Read the model definition and answer for the solid it produces. Units are mm, in the model's axes. A direction names the side the tool comes from. Give positions to 0.01 mm unless a question says otherwise; leave off trailing zeros. Order: outer loops, then holes, each group sorted by start corner. A loop starts at its lowest first (then second) coordinate and runs counter-clockwise, first axis right, second up. Notation, with made-up numbers: (20, 71) -> (61, 71) arc R21 cw to (61, 103) -> close; hole circle Ø7 at (64.5, -34). An arc over 180 degrees is marked (long way). Answer as CSV lines item,"result". Start each with the question number.
1) Straight lines are drawn through the part: L1, parallel to Z at x = 19.5, y = 1.7; L2, parallel to Z at x = 19.25, y = 1.35; L3, parallel to X at y = 0.4, z = 3. For each, find the intervals that lie inside material, in ascending order. Write a range as from..to.
2) Find section B-B (z = 2). Determine the outline of the cut face in (x, y), and give its area (3 significant figures).
3) For faces 1 (the face through (14, 2, 0)), 2 (the face through (19, 2, -3)), 3 (the face through (9, 1, 2.5)), determine the directions among +Z, -Z, +X, -X, +Y, -Y from which every point of the face is accessible in a straight line to the end or side of a thin tool.
4) Flat-ended cylindrical pins translate along their axes: pin 1 Ø1.5 at (x, y) = (10, 1.5) entering from -Z; pin 2 Ø0.6 at (x, y) = (11.5, 1) entering from -Z; pin 3 Ø0.9 at (y, z) = (2, -2) entering from +X. Find the tip coordinate at first contact, or state that the pin passes through.
5) Find section C-C (x = 5.75). Determine the outline of the cut face in (y, z).
6) Find section D-D (y = 1.8). State how many separate pieces and enclosed holes the cut face has, and give its area (3 significant figures).
7) The mould has two halves that part along X. Classify faces 4 (the face through (8.328, 1, 4)), 5 (the face through (13, 1, 2.5)), 6 (the face through (15, 0, 12)), 7 (the face through (24.4, 1.52, 26.43)): +X half, -X half, draft (parallel to the pull), parting line (faces both ways), or undercut.
8) Find section A-A (z = 8). Determine the outline of the cut face in (x, y), and give its area (3 significant figures).
```python
from build123d import *

# Parameters (mm, degrees)
SKETCH_1_W          = 25
SKETCH_1_H          = 5
EXTRUDE_1_DEPTH     = 24
SKETCH_2_W          = 5
SKETCH_2_H          = 5
SKETCH_2_W_2        = 8
EXTRUDE_2_DEPTH     = 3
CUT_EXTRUDE_2_DEPTH = 5
EXTRUDE_3_DEPTH     = 5
FILLET_1_R          = 5
FILLET_2_R          = 2
CUT_EXTRUDE_4_DEPTH = 2
CUT_EXTRUDE_5_DEPTH = 3
SKETCH_9_R          = 2
CUT_EXTRUDE_6_DEPTH = 3
SKETCH_10_W         = 7
SKETCH_10_H         = 3
CUT_EXTRUDE_7_DEPTH = 3


with BuildPart() as part:
    # 草图1 → 凸台-拉伸1 (new body)
    with BuildSketch(Plane.XY):
        with Locations((12.5, 2.5)):
            Rectangle(SKETCH_1_W, SKETCH_1_H)
    extrude(amount=EXTRUDE_1_DEPTH)

    # 草图2 → 凸台-拉伸2 (add)
    with BuildSketch(Plane(origin=(0, 0, 0), x_dir=(-1, 0, 0), z_dir=(0, 0, -1))):
        with Locations((-4.5, 2.5)):
            Rectangle(SKETCH_2_W, SKETCH_2_H)
        with Locations((-19, 2.5)):
            Rectangle(SKETCH_2_W_2, SKETCH_2_H)
    extrude(amount=EXTRUDE_2_DEPTH)

    # 草图3 → 切除-拉伸2 (cut)
    with BuildSketch(Plane.XZ):
        Polygon((12.5, 24), (0, 24), (0, 0), align=None)
    extrude(amount=-CUT_EXTRUDE_2_DEPTH, mode=Mode.SUBTRACT)

    # 草图4 → 凸台-拉伸3 (add)
    with BuildSketch(Plane.XZ):
        Polygon((12.5, 24), (25, 24), (25, 27), (14.0625, 27), align=None)
    extrude(amount=-EXTRUDE_3_DEPTH)

    # 圆角1
    fillet_1_edges = [part.edges().sort_by_distance(p)[0] for p in [
        (14.0625, 2.5, 27),
    ]]
    fillet(fillet_1_edges, radius=FILLET_1_R)

    # 圆角2
    fillet_2_edges = [part.edges().sort_by_distance(p)[0] for p in [
        (25, 2.5, 27),
    ]]
    fillet(fillet_2_edges, radius=FILLET_2_R)

    # 草图7 → 切除-拉伸4 (cut)
    with BuildSketch(Plane(origin=(0, 5, 0), x_dir=(1, 0, 0), z_dir=(0, 1, 0))):
        with BuildLine():
            Line((17.09585797, -27), (23, -27))
            ThreePointArc((23, -27), (24.414213562, -26.414213562), (25, -25))
            Line((25, -25), (25, 0))
            Line((25, 0), (23, 0))
            Line((23, 0), (23, 3))
            Line((23, 3), (15, 3))
            Line((15, 3), (15, 0))
            Line((15, 0), (7, 0))
            Line((7, 0), (7, 3))
            Line((7, 3), (2, 3))
            Line((2, 3), (2, 0))
            Line((2, 0), (0, 0))
            Line((0, 0), (12.661287549, -24.309672094))
            ThreePointArc((12.661287549, -24.309672094), (14.502439422, -26.274831018), (17.09585797, -27))
        make_face()
    extrude(amount=-CUT_EXTRUDE_4_DEPTH, mode=Mode.SUBTRACT)

    # 草图8 → 切除-拉伸5 (cut)
    with BuildSketch(Plane(origin=(38.221211183, 0, -111.620742166), x_dir=(0, 0, -1), z_dir=(0, -1, 0))):
        with BuildLine():
            Line((-114.120742166, -28.543003338), (-111.620742166, -28.543003338))
            Line((-111.620742166, -28.543003338), (-111.620742166, -25.743003338))
            Line((-111.620742166, -25.743003338), (-114.120742166, -25.743003338))
            Line((-114.120742166, -25.743003338), (-114.120742166, -24.693003338))
            ThreePointArc((-114.120742166, -24.693003338), (-114.208610132, -24.480871304), (-114.420742166, -24.393003338))
            Line((-114.420742166, -24.393003338), (-116.320742166, -24.393003338))
            ThreePointArc((-116.320742166, -24.393003338), (-116.5328742, -24.480871304), (-116.620742166, -24.693003338))
            Line((-116.620742166, -24.693003338), (-116.620742166, -25.793003338))
            Line((-116.620742166, -25.793003338), (-116.820742166, -25.793003338))
            ThreePointArc((-116.820742166, -25.793003338), (-117.0328742, -25.880871304), (-117.120742166, -26.093003338))
            Line((-117.120742166, -26.093003338), (-117.120742166, -28.193003338))
            ThreePointArc((-117.120742166, -28.193003338), (-117.0328742, -28.405135373), (-116.820742166, -28.493003338))
            Line((-116.820742166, -28.493003338), (-116.620742166, -28.493003338))
            Line((-116.620742166, -28.493003338), (-116.620742166, -29.593003338))
            ThreePointArc((-116.620742166, -29.593003338), (-116.5328742, -29.805135373), (-116.320742166, -29.893003338))
            Line((-116.320742166, -29.893003338), (-114.420742166, -29.893003338))
            ThreePointArc((-114.420742166, -29.893003338), (-114.208610132, -29.805135373), (-114.120742166, -29.593003338))
            Line((-114.120742166, -29.593003338), (-114.120742166, -28.543003338))
        make_face()
    extrude(amount=-CUT_EXTRUDE_5_DEPTH, mode=Mode.SUBTRACT)

    # 草图9 → 切除-拉伸6 (cut)
    with BuildSketch(Plane(origin=(38.221211183, 0, -111.620742166), x_dir=(0, 0, -1), z_dir=(0, -1, 0))):
        with Locations((-130.672383052, -17.574261788)):
            Circle(SKETCH_9_R)
    extrude(amount=-CUT_EXTRUDE_6_DEPTH, mode=Mode.SUBTRACT)

    # 草图10 → 切除-拉伸7 (cut)
    with BuildSketch(Plane(origin=(38.221211183, 0, -111.620742166), x_dir=(0, 0, -1), z_dir=(0, -1, 0))):
        with Locations((-122.120742166, -18.681849587)):
            Rectangle(SKETCH_10_W, SKETCH_10_H)
    extrude(amount=-CUT_EXTRUDE_7_DEPTH, mode=Mode.SUBTRACT)


solid = part.part
```
Findings below:
1,L1,"-3..7, 14..17.41, 20.69..27"
1,L2,"-3..7, 14..17.62, 20.48..27"
1,L3,"1.56..8.33, 13.83..25"
2,outline,"(1.04, 0) -> (9.68, 0) -> (9.68, 3) -> (1.04, 3) -> close; (12.48, 0) -> (25, 0) -> (25, 3) -> (12.48, 3) -> close"
2,area,"63.5 mm²"
3,face 1,"-Z, +Y, -Y"
3,face 2,"-Z, +X, -X, +Y, -Y"
3,face 3,"+Y, -Y"
4,pin 1,"z = 0"
4,pin 2,"z = 5.5"
4,pin 3,"x = 23"
5,outline,"(0, -3) -> (3, -3) -> (3, 11.04) -> (0, 11.04) -> close"
6,separate pieces,"1"
6,enclosed holes,"2"
6,area,"466 mm²"
7,face 4,"undercut"
7,face 5,"undercut"
7,face 6,"draft"
7,face 7,"+X half"
8,outline,"(4.17, 0) -> (18.04, 0) -> (18.04, 3) -> (4.17, 3) -> close; (21.04, 0) -> (25, 0) -> (25, 3) -> (21.04, 3) -> close"
8,area,"53.5 mm²"
